The drawing under review shows one solid part. Ordinate dimensions are in mm from its lowest x, y, z. Round coordinates to 2 decimals unless told otherwise and drop trailing zeros. Order: outer loops, then holes, each group sorted by start corner. A loop starts at its lowest first (then second) coordinate and runs counter-clockwise, first axis right, second up. Notation, with made-up numbers: (-11.5, -3) - (41.5, -3) arc R23 ccw to (41.5, 11) - close; hole circle Ø5 at (53.5, 46.25). An arc over 180 degrees is marked (long way). One line per question, with ' | ' between items.
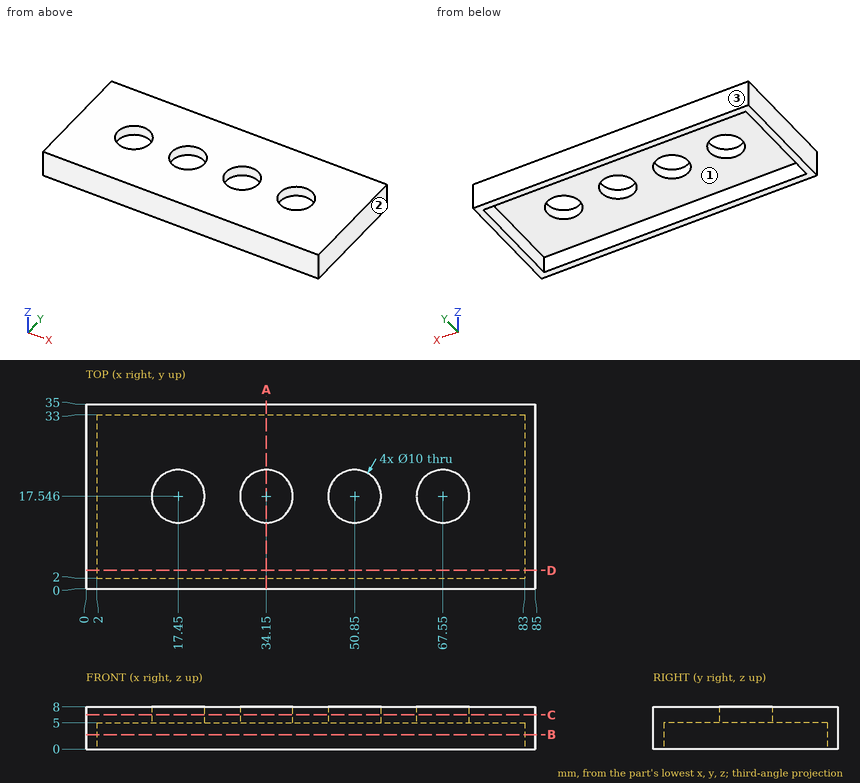
(1) For probe 1 along X at (y, z) = (16.5, 2); probe 2 along Y at (x, z) = (57, 1.75); probe 3 along Y at (x, z) = (34.15, 7.1), list the stretches that pass through material, from the lowest coordinate up. Write a range as [from, to].
Output values:
probe 1: [0, 2], [83, 85] | probe 2: [0, 2], [33, 35] | probe 3: [0, 12.55], [22.55, 35]
(2) We need section C-C on z = 6.5. State the section outline as (x, y) points.
Output values:
outline: (0, 0) - (85, 0) - (85, 35) - (0, 35) - close; hole circle Ø10 at (17.45, 17.55); hole circle Ø10 at (34.15, 17.55); hole circle Ø10 at (50.85, 17.55); hole circle Ø10 at (67.55, 17.55)
(3) We need section D-D on y = 3.5. State the section outline as (x, z) points.
Output values:
outline: (0, 0) - (2, 0) - (2, 5) - (83, 5) - (83, 0) - (85, 0) - (85, 8) - (0, 8) - close
(4) Insertion check: pin 1 (15.5 mm diameter, centred on x = 32.5, y = 11.5, fed in from -Z). The pin has a flat end and moves straight along its axis. Give the tip position at first contact, or say it passes through.
Output values:
pin 1: z = 5
(5) We need section A-A on x = 34.15. State the section outline as (y, z) points.
Output values:
outline: (0, 0) - (2, 0) - (2, 5) - (12.55, 5) - (12.55, 8) - (0, 8) - close; (22.55, 5) - (33, 5) - (33, 0) - (35, 0) - (35, 8) - (22.55, 8) - close
(6) We need section B-B on z = 2.75. State the section outline as (x, y) points, plus the area to 3 significant figures.
Output values:
outline: (0, 0) - (85, 0) - (85, 35) - (0, 35) - close; hole (2, 2) - (83, 2) - (83, 33) - (2, 33) - close | area: 464 mm^2
(7) Mouldability with a two-part tool opening along Y and no side actions: class the marked faces 1, 2 and 3 as released by +Y, released by -Y, zero draft, split by the parting line, or undercut.
Output values:
face 1: undercut | face 2: zero draft | face 3: released by +Y
